```python
from build123d import *

# Parameters (mm, degrees)
CROQUIS1_W              = 80
CROQUIS1_H              = 12
SALIENTE_EXTRUIR1_DEPTH = 12
CORTAR_EXTRUIR1_DEPTH   = 12


with BuildPart() as part:
    # Croquis1 → Saliente-Extruir1 (new body)
    with BuildSketch(Plane(origin=(0, 0, 0), x_dir=(1, 0, 0), z_dir=(0, 1, 0))):
        with Locations((40, 6)):
            Rectangle(CROQUIS1_W, CROQUIS1_H)
    extrude(amount=SALIENTE_EXTRUIR1_DEPTH)

    # Croquis2 → Cortar-Extruir1 (cut)
    with BuildSketch(Plane.XY):
        with BuildLine():
            ThreePointArc((40, 2.81412174), (46.163496931, 6), (40, 9.18587826))
            ThreePointArc((40, 9.18587826), (33.836503069, 6), (40, 2.81412174))
        make_face()
    extrude(amount=-CORTAR_EXTRUIR1_DEPTH, mode=Mode.SUBTRACT)


solid = part.part
```
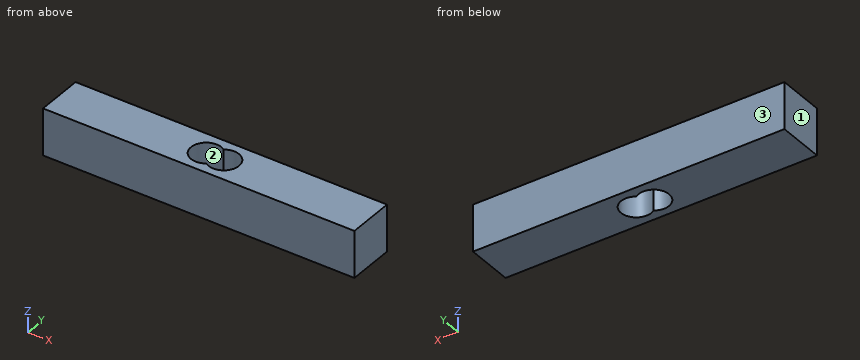
Geometry: final body of the model. Coordinates: model frame, mm. Face numbers are marked on the shaded views. Round coordinates to 2 decimals unless told otherwise and drop trailing zeros. Loops run counter-clockwise (first coordinate to the right, second up) from the corner with the lowest first, then second, coordinate; pieces in that order, holes last.
Item 1: Contact query for a flat-ended pin moving along its axis: P1, Ø4, axis at x = 41, y = 3, coming from the +Z side. Output: stop coordinate, or through.
Checked values:
P1: stops at z = 0
Item 2: Line query: L1, parallel to Y at x = 42, z = -10.75; L2, parallel to X at y = 4.75, z = -11; L3, parallel to Y at x = 45, z = -3.75. Output: solid intervals per line, ascending.
Checked values:
L1: y = 0 to 2.1, 9.9 to 12
L2: x = 0 to 34.04, 45.96 to 80
L3: y = 0 to 3.22, 8.78 to 12
Item 3: Mould query, pull axis Y, two halves, no side actions, for the marked faces 1, 2 and 3. Classes: released by +Y, released by -Y, zero draft, split by the parting line, or undercut.
Checked values:
face 1: zero draft
face 2: undercut
face 3: released by +Y
Item 4: Section A-A, the plane y = 6. Output: boundary loops of the cut face in (x, z), plus the area to 3 significant figures.
Checked values:
outline: (0, -12) - (33.84, -12) - (33.84, 0) - (0, 0) - close; (46.16, -12) - (80, -12) - (80, 0) - (46.16, 0) - close
area: 812 mm2
Item 5: Section B-B, the plane x = 41. Output: boundary loops of the cut face in (y, z).
Checked values:
outline: (0, -12) - (2.3, -12) - (2.3, 0) - (0, 0) - close; (9.7, -12) - (12, -12) - (12, 0) - (9.7, 0) - close
Item 6: Section C-C, the plane z = -10. Output: boundary loops of the cut face in (x, y).
Checked values:
outline: (0, 0) - (80, 0) - (80, 12) - (0, 12) - close; hole (40, 2.81) arc R3.91 ccw (long way) to (40, 9.19) arc R3.91 ccw (long way) to start
